Autodesk Inventor part; units mm, degrees
ref_plane "YZ Plane" through (0, 0, 0) normal (1, 0, 0) x (0, 1, 0)
ref_plane "XZ Plane" through (0, 0, 0) normal (0, 1, 0) x (-1, 0, 0)
ref_plane "XY Plane" through (0, 0, 0) normal (0, 0, 1) x (1, 0, 0)
sketch "Sketch1" plane through (0, 0, 0) normal (1, 0, 0) x (0, 1, 0)
  line L0 (-27, 60) -> (27, 60)
  line L1 (27, 60) -> (27, -60)
  line L2 (27, -60) -> (-27, -60)
  line L3 (-27, -60) -> (-27, 60)
  line L4 (-27, 60) -> (27, -60) construction
  line L5 (27, 60) -> (-27, -60) construction
  point P0 (0, 0)
  dimension "d0" = 54
  dimension "d1" = 120
extrude "Extrusion1" add sketch "Sketch1" along normal mid plane 3.175
sketch "Sketch2" plane through (1.5875, 0, 0) normal (1, 0, 0) x (0, 0, -1)
  circle A0 centre (-48, -17) radius 2.5 construction
  line L0 (-60, -27) -> (60, -27) construction
  circle A1 centre (-54, -23) radius 2
  circle A2 centre (-42, -23) radius 2
  circle A3 centre (-42, -11) radius 2
  circle A4 centre (-54, -11) radius 2
  line L1 (0, 27) -> (0, -27) construction
  line L2 (60, 27) -> (-60, 27) construction
  line L3 (-60, 27) -> (-60, -27) construction
  line L4 (60, -27) -> (60, 27) construction
  line L5 (-60, 0) -> (60, 0) construction
  circle A5 centre (54, -23) radius 2
  circle A6 centre (42, -23) radius 2
  circle A7 centre (42, -11) radius 2
  circle A8 centre (54, -11) radius 2
  circle A9 centre (-54, 23) radius 2
  circle A10 centre (-42, 23) radius 2
  circle A11 centre (-42, 11) radius 2
  circle A12 centre (-54, 11) radius 2
  circle A13 centre (54, 11) radius 2
  circle A14 centre (42, 11) radius 2
  circle A15 centre (54, 23) radius 2
  circle A16 centre (42, 23) radius 2
  point P0 (0, 0)
  dimension "d4" = 5
  dimension "d5" = 48
  dimension "d6" = 10
  dimension "d7" = 4
  dimension "d8" = 6
  dimension "d9" = 6
  dimension "d12" = 360
extrude "Extrusion2" cut sketch "Sketch2" against normal through all
sketch "Sketch4" plane through (1.5875, 0, 0) normal (1, 0, 0) x (0, 0, -1)
  circle A0 centre (0, 6) radius 18
  circle A1 centre (-28, 22) radius 2
  line L0 (0, 24) -> (0, -12) construction
  line L1 (60, 27) -> (-60, 27) construction
  line L2 (-18, 6) -> (18, 6) construction
  circle A2 centre (-16, 22) radius 2
  circle A3 centre (28, 22) radius 2
  circle A4 centre (-28, -10) radius 2
  circle A5 centre (28, -10) radius 2
  circle A6 centre (-16, -10) radius 2
  circle A7 centre (16, -10) radius 2
  circle A8 centre (16, 22) radius 2
  point P0 (0, 0)
  dimension "d30" = 36
  dimension "d31" = 6
  dimension "d32" = 4
  dimension "d33" = 28
  dimension "d34" = 16
  dimension "d35" = 4
  dimension "d36" = 16
  dimension "d37" = 16
  dimension "d40" = 360
extrude "Extrusion4" cut sketch "Sketch4" against normal through all
properties part number "TurretMotorCase_SidePlate"
Can you work these out from the model? Positions are in its coordinate system, mm. Give positions to 0.01 mm unless a question says otherwise; leave off trailing zeros. Loops run counter-clockwise (first coordinate to the right, second up) from the corner with the lowest first, then second, coordinate; pieces in that order, holes last. Notation, with made-up numbers: M -34,10.25 L -29,10.25 A21 cw -29,18.25 Z; hole C 83,-16.5 d7. An arc over 180 degrees is marked long. One line per question, with ' | ' between items. Start each with the question number.
Q1. If we section it at B-B (y = -23): Please give me the cut outline in (x, z), plus the area to 3 significant figures.
Q2. If we section it at C-C (z = -54): Please give me the cut outline in (x, y), plus the area to 3 significant figures.
Q3. If we section it at D-D (z = -28): Please give me the cut outline in (x, y).
Q4. If we mould it in two halves opening along Z, with no side actions, what happens to faces 1 (the flat face through (0, 0, 60)), 2 (the cylindrical face through (0, 21.8, -52.4)), 3 (the flat face through (-1.588, -12.4, 0.8))? For each: +Z half, -Z half, draft (parallel to the pull), parting line (faces both ways), or undercut.
Q5. If we section it at A-A (x = 0.7): State how many separate pieces and enclosed holes the cut face has, plus the area to 3 significant figures.
Q6. If I drill on line 1 (Y direction, x = -0.4, z = 28); line 2 (Y direction, x = 1.4, z = -54); line 3 (Y direction, x = -0.55, z = 42.5), over which ranges is the centre line in solid material (lowest first)? Write a range as from..to.
Computed:
1) outline: M -1.59,-60 L 1.59,-60 L 1.59,-56 L -1.59,-56 Z; M -1.59,-52 L 1.59,-52 L 1.59,-44 L -1.59,-44 Z; M -1.59,-40 L 1.59,-40 L 1.59,40 L -1.59,40 Z; M -1.59,44 L 1.59,44 L 1.59,52 L -1.59,52 Z; M -1.59,56 L 1.59,56 L 1.59,60 L -1.59,60 Z | area: 330 mm²
2) outline: M -1.59,-27 L 1.59,-27 L 1.59,-25 L -1.59,-25 Z; M -1.59,-21 L 1.59,-21 L 1.59,-13 L -1.59,-13 Z; M -1.59,-9 L 1.59,-9 L 1.59,9 L -1.59,9 Z; M -1.59,13 L 1.59,13 L 1.59,21 L -1.59,21 Z; M -1.59,25 L 1.59,25 L 1.59,27 L -1.59,27 Z | area: 121 mm²
3) outline: M -1.59,-27 L 1.59,-27 L 1.59,-12 L -1.59,-12 Z; M -1.59,-8 L 1.59,-8 L 1.59,20 L -1.59,20 Z; M -1.59,24 L 1.59,24 L 1.59,27 L -1.59,27 Z
4) face 1: +Z half | face 2: undercut | face 3: draft
5) separate pieces: 1 | enclosed holes: 25 | area: 5,160 mm²
6) line 1: y = -27..-12, -8..20, 24..27 | line 2: y = -27..-25, -21..-13, -9..9, 13..21, 25..27 | line 3: y = -27..-24.94, -21.06..-12.94, -9.06..9.06, 12.94..21.06, 24.94..27
